For this review, take the finished solid that the model builds, in its own axes (mm). Give positions to 0.01 mm unless a question says otherwise; leave off trailing zeros. Write each loop counter-clockwise with the first axis right and the second up, starting at its lowest first coordinate (ties: lowest second). Pieces come first, ordered by that corner, then holes. Notation, with made-up numbers: (50.5, 79) -> (93.5, 79) arc R19 ccw to (93.5, 93) -> close; hole circle Ø3 at (-15.5, -16). An arc over 180 degrees is marked (long way). Answer as CSV lines item,"result".
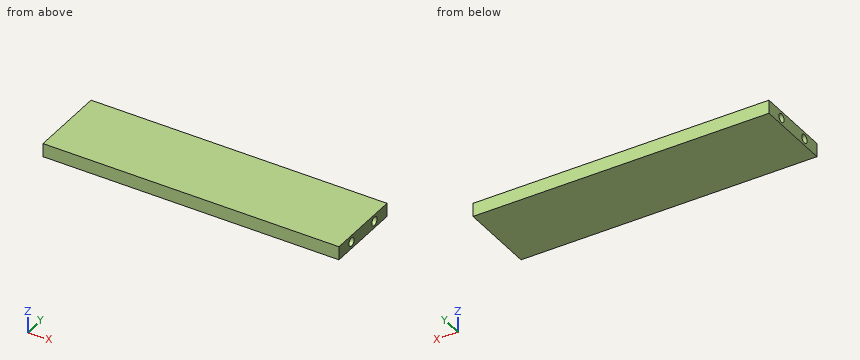
```python
from build123d import *

# Parameters (mm, degrees)
ESBO_O1_W                = 88.01
ESBO_O1_H                = 23
RESSALTO_EXTRUS_O1_DEPTH = 4
ESBO_O2_R                = 1.25
CORTE_EXTRUS_O1_DEPTH    = 10
ESBO_O3_R                = 1.25
CORTE_EXTRUS_O2_DEPTH    = 10


with BuildPart() as part:
    # Esboço1 → Ressalto-extrusão1 (new body)
    with BuildSketch(Plane.XY):
        with Locations((44.005, -11.5)):
            Rectangle(ESBO_O1_W, ESBO_O1_H)
    extrude(amount=RESSALTO_EXTRUS_O1_DEPTH)

    # Esboço2 → Corte-extrusão1 (cut)
    with BuildSketch(Plane.ZY):
        with Locations((2, -6)):
            Circle(ESBO_O2_R)
        with Locations((2, -17)):
            Circle(ESBO_O2_R)
    extrude(amount=-CORTE_EXTRUS_O1_DEPTH, mode=Mode.SUBTRACT)

    # Esboço3 → Corte-extrusão2 (cut)
    with BuildSketch(Plane(origin=(88.01, 0, 0), x_dir=(0, 0, -1), z_dir=(1, 0, 0))):
        with Locations((-2, -6)):
            Circle(ESBO_O3_R)
        with Locations((-2, -17)):
            Circle(ESBO_O3_R)
    extrude(amount=-CORTE_EXTRUS_O2_DEPTH, mode=Mode.SUBTRACT)


solid = part.part
```
Q1. To check wall thickness, follow probe 1 along Y at (x, z) = (84.75, 2); probe 2 along Y at (x, z) = (84, 1.4). State the ranges of each line that lie inside material, in increasing order. Write a range as [from, to].
Answer block:
probe 1,"y = [-23, -18.25], [-15.75, -7.25], [-4.75, 0]"
probe 2,"y = [-23, -18.1], [-15.9, -7.1], [-4.9, 0]"
Q2. Clearance check with a flat-ended pin moving along its axis: pin 1 (0.8 mm diameter, centred on y = -5.5, z = 1.5, fed in from +X). State where the tip first meets the part, or that it passes through.
Answer block:
pin 1,"stops at x = 78.01"
Q3. Add section B-B (y = -6). Write out the cut boundary in (x, z).
Answer block:
outline,"(0, 0) -> (88.01, 0) -> (88.01, 0.75) -> (78.01, 0.75) -> (78.01, 3.25) -> (88.01, 3.25) -> (88.01, 4) -> (0, 4) -> (0, 3.25) -> (10, 3.25) -> (10, 0.75) -> (0, 0.75) -> close"
Q4. Add section A-A (z = 2). Write out the cut boundary in (x, y), plus the area to 3 significant figures.
Answer block:
outline,"(0, -23) -> (88.01, -23) -> (88.01, -18.25) -> (78.01, -18.25) -> (78.01, -15.75) -> (88.01, -15.75) -> (88.01, -7.25) -> (78.01, -7.25) -> (78.01, -4.75) -> (88.01, -4.75) -> (88.01, 0) -> (0, 0) -> (0, -4.75) -> (10, -4.75) -> (10, -7.25) -> (0, -7.25) -> (0, -15.75) -> (10, -15.75) -> (10, -18.25) -> (0, -18.25) -> close"
area,"1,920 mm2"
